```python
from build123d import *

# Parameters (mm, degrees)
F0_W     = 20
F0_H     = 5
F0_W_2   = 10
F0_H_2   = 3.8665379398
F0_H_3   = 20
F0_R     = 1.6
F1_DEPTH = 4
F2_DEPTH = 20
F3_DEPTH = 66
F4_R     = 1.5
F6_DEPTH = 3.5
F7_DEPTH = 3.5
F8_DEPTH = 25


# Not quite as in the source:
# - an extrude ends at something that could not be found from the text; its depth is read off the source's solid


with BuildPart() as f1:
    # F0 (on Right) → F1 (new body)
    with BuildSketch(Plane.YZ):
        Polygon((3.6049238205, -6.8721993268), (3.6049238205, 13.1278006732), (-16.3950761795, 13.1278006732), (-16.3950761795, 6.6331364214), (-6.3950761795, 6.6331364214), (-6.3950761795, 2.7665984817), (-16.3950761795, 2.7665984817), (-16.3950761795, -6.8721993268), align=None)
        with Locations((-6.3950761795, -9.3721993268)):
            Rectangle(F0_W, F0_H)
        with Locations((-11.3950761795, 4.6998674516)):
            Rectangle(F0_W_2, F0_H_2)
        with Locations((-6.3950761795, -21.8721993268)):
            Rectangle(F0_W, F0_H_3)
        with Locations((-11.7450761795, -17.3721993268)):
            Circle(F0_R, mode=Mode.SUBTRACT)
        with Locations((-1.0450761795, -17.3721993268)):
            Circle(F0_R, mode=Mode.SUBTRACT)
    extrude(amount=F1_DEPTH)

    # F0 (on Right) → F2 (join)
    with BuildSketch(Plane.YZ):
        with Locations((-6.3950761795, -9.3721993268)):
            Rectangle(F0_W, F0_H)
    extrude(amount=F2_DEPTH)

    # F0 (on Right) → F3 (cut, through all)
    with BuildSketch(Plane.YZ):
        with Locations((-1.0450761795, -17.3721993268)):
            Circle(F0_R)
    extrude(amount=-F3_DEPTH, mode=Mode.SUBTRACT)

    # F4
    f4_edges = [f1.edges().sort_by_distance(p)[0] for p in [
        (0, 3.604924, -9.372199),
        (0, -6.395076, 13.127801),
        (0, -16.395076, -9.372199),
        (0, -6.395076, -31.872199),
        (2, 3.604924, 13.127801),
        (2, 3.604924, -31.872199),
        (2, -16.395076, 13.127801),
        (2, -16.395076, -31.872199),
        (12, -16.395076, -6.872199),
        (12, 3.604924, -6.872199),
        (20, -6.395076, -6.872199),
        (20, 3.604924, -9.372199),
        (20, -16.395076, -9.372199),
    ]]
    fillet(f4_edges, radius=F4_R)

    # F5 (on face) → F6 (join)
    with BuildSketch(Plane(origin=(0, 0, -11.8721993268), x_dir=(1, 0, 0), z_dir=(0, 0, -1))):
        with BuildLine():
            Line((15.1547100395, 8.9950761795), (20, 8.9950761795))
            Line((20, 8.9950761795), (20, 14.8950761795))
            ThreePointArc((20, 14.8950761795), (19.686066448, 15.8133606567), (18.8756714919, 16.3472713903))
            Line((18.8756714919, 16.3472713903), (15.1547100395, 16.3472713903))
            Line((15.1547100395, 16.3472713903), (15.1547100395, 8.9950761795))
        make_face()
        with BuildLine():
            Line((20, -2.1049238205), (20, 3.7950761795))
            Line((20, 3.7950761795), (15.1547100395, 3.7950761795))
            Line((15.1547100395, 3.7950761795), (15.1547100395, -3.5571190313))
            Line((15.1547100395, -3.5571190313), (18.8756714919, -3.5571190313))
            ThreePointArc((18.8756714919, -3.5571190313), (19.686066448, -3.0232082977), (20, -2.1049238205))
        make_face()
    extrude(amount=F6_DEPTH)

    # F5 (on face) → F7 (join)
    with BuildSketch(Plane(origin=(0, 0, -11.8721993268), x_dir=(1, 0, 0), z_dir=(0, 0, -1))):
        with BuildLine():
            Line((15.1547100395, 8.9950761795), (20, 8.9950761795))
            Line((20, 8.9950761795), (20, 14.8950761795))
            ThreePointArc((20, 14.8950761795), (19.686066448, 15.8133606567), (18.8756714919, 16.3472713903))
            Line((18.8756714919, 16.3472713903), (15.1547100395, 16.3472713903))
            Line((15.1547100395, 16.3472713903), (15.1547100395, 8.9950761795))
        make_face()
    extrude(amount=F7_DEPTH)

    # F5 (on face) → F8 (cut)
    with BuildSketch(Plane(origin=(0, 0, -11.8721993268), x_dir=(1, 0, 0), z_dir=(0, 0, -1))):
        Polygon((20, 3.7950761795), (20, 8.9950761795), (15.1547100395, 8.9950761795), (9.3279955909, 8.9950761795), (9.3279955909, 3.7950761795), (15.1547100395, 3.7950761795), align=None)
    extrude(amount=-F8_DEPTH, mode=Mode.SUBTRACT)


solid = f1.part
```
For this review, take the finished solid that the model builds, in its own axes (mm). A direction names the side the tool comes from. Coordinates: 2 decimals unless noted, no trailing zeros. Loops run counter-clockwise (first coordinate to the right, second up) from the corner with the lowest first, then second, coordinate; pieces in that order, holes last.
1. Add section B-B, the plane z = -14. Give the boundary of the cut face in (x, y), then the cut area to 3 significant figures.
2. For line 1 (Y direction, x = 17.25, z = -11); line 2 (X direction, y = -14.5, z = -19.5); line 3 (Z direction, x = 9.5, y = -1.25), list the stretches that pass through material, from the lowest coordinate up.
3. Add section C-C, the plane y = -7.5. Give the boundary of the cut face in (x, z), then the cut area to 3 significant figures.
4. Mouldability with a two-part tool opening along X and no side actions: class faces 6 (the flat face through (15.155, -13, -14)), 7 (the cylindrical face through (2.77, -15.97, -31.42)), 8 (the cylindrical face through (19.55, -11.9, -7.3)) as +X half, -X half, draft (parallel to the pull), parting line (faces both ways), or undercut.
5. For faces 1 (the flat face through (18, -13, -15.372)), 2 (the flat face through (3, -6, 13.128)), 3 (the flat face through (4, -7, -22)), 4 (the flat face through (17, 3.557, -14)), 5 (the flat face through (17, -16.347, -14)), list the 3-axis set-ups (+Z, -Z, +X, -X, +Y, -Y) from which the entire face can be reached by the end or side of a thin tool; tool diameter is ignored.
6. Add section D-D, the plane x = 2.25. Give the boundary of the cut face in (y, z), then the cut area to 3 significant figures.
7. Insertion check: P1, Ø7, axis at x = 14, y = -2.5, coming from the +Z side; P2, Ø1, axis at x = 10.5, y = -10.5, coming from the -Z side; P3, Ø3.5, axis at y = -1.05, z = -17.37, coming from the +X side; P4, Ø2.5, axis at y = -11.75, z = -17.37, coming from the -X side. Each pin has a flat end and moves straight along its axis. Give the tip position at first contact, or say it passes through.
8. Add section A-A, the plane x = 16.75. Give the boundary of the cut face in (y, z).
Result:
1. outline: (0, -14.9) arc R1.5 ccw to (1.5, -16.4) - (4, -16.4) - (4, 3.6) - (1.5, 3.6) arc R1.5 ccw to (0, 2.1) - close; (15.15, -16.35) - (18.88, -16.35) arc R1.5 ccw to (20, -14.9) - (20, -9) - (15.15, -9) - close; (15.15, -3.8) - (20, -3.8) - (20, 2.1) arc R1.5 ccw to (18.88, 3.56) - (15.15, 3.56) - close
1. area: 149 mm2
2. line 1: y = -16.4 to -9, -3.8 to 3.6
2. line 2: x = 0 to 4
2. line 3: z = -11.87 to -6.87
3. outline: (0, -30.37) arc R1.5 ccw to (1.5, -31.87) - (4, -31.87) - (4, -11.87) - (9.33, -11.87) - (9.33, -6.87) - (4, -6.87) - (4, 13.13) - (1.5, 13.13) arc R1.5 ccw to (0, 11.63) - close
3. area: 206 mm2
4. face 6: undercut
4. face 7: draft
4. face 8: +X half
5. face 1: -Z, +X, +Y, -Y
5. face 2: +Z, +X, -X, +Y, -Y
5. face 3: -Z, +Y, -Y
5. face 4: -Z, +X, +Y
5. face 5: -Z, +X, -Y
6. outline: (-16.4, -30.37) arc R1.5 ccw to (-14.9, -31.87) - (2.1, -31.87) arc R1.5 ccw to (3.6, -30.37) - (3.6, 11.63) arc R1.5 ccw to (2.1, 13.13) - (-14.9, 13.13) arc R1.5 ccw to (-16.4, 11.63) - close; hole circle Ø3.2 at (-11.75, -17.37); hole circle Ø3.2 at (-1.05, -17.37)
6. area: 882 mm2
7. P1: stops at z = -6.87
7. P2: stops at z = -11.87
7. P3: stops at x = 4
7. P4: passes through
8. outline: (-16.4, -11.87) - (-16.35, -11.87) - (-16.35, -15.37) - (-9, -15.37) - (-9, -6.87) - (-14.9, -6.87) arc R1.5 ccw to (-16.4, -8.37) - close; (-3.8, -15.37) - (3.56, -15.37) - (3.56, -11.87) - (3.6, -11.87) - (3.6, -8.37) arc R1.5 ccw to (2.1, -6.87) - (-3.8, -6.87) - close
